The model under review builds one solid part; all positions refer to its coordinate system, in mm. Coordinates: 2 decimals unless noted, no trailing zeros. Loops run counter-clockwise (first coordinate to the right, second up) from the corner with the lowest first, then second, coordinate; pieces in that order, holes last. Notation, with made-up numbers: (57.25, 52.25) - (111.25, 52.25) arc R30 cw to (111.25, 90.25) - close; hole circle Ø3 at (11.25, 49). An arc over 180 degrees is marked (long way). Answer in a Markdown table with one row per item. Add a question column.
(1) For P1, Ø1.5, axis at y = 1, z = -30.5, coming from the +X side; P2, Ø1, axis at x = -1.5, y = 2.5, coming from the -Z side, all flat-tipped, find the tip position at first contact; note any pin that passes through.
(2) We need section D-D on x = 0. Write out the cut boundary in (y, z), plus the area to 3 significant figures.
(3) We need section B-B on y = 1.7. Give the number of separate pieces and of enclosed holes in the cut face, plus the area to 3 significant figures.
(4) We need section C-C on z = 9. Write out the cut boundary in (x, y).
(5) For line 1 along X through (y, z) = (2.1, 0); line 2 along X through (y, z) = (1.9, 30); line 3 along Z through (x, y) = (-32, 1.55), list the stretches that pass through material, from the lowest coordinate up.
(6) Mouldability with a two-part tool opening along X and no side actions: class faces 1 (the cylindrical face through (15.02, 1.48, 47.69)), 2 (the cylindrical face through (-20.196, 1.479, -0.488)), 3 (the flat face through (12, 3, -1)) as +X half, -X half, draft (parallel to the pull), parting line (faces both ways), or undercut.
(7) We need section A-A on x = 30. Write out the cut boundary in (y, z).
from build123d import *

# Parameters (mm, degrees)
SKETCH_1_R          = 50
EXTRUDE_2_DEPTH     = 3
SKETCH_3_R          = 2.25
CUT_EXTRUDE_1_DEPTH = 71.774289117
SKETCH_4_R          = 11
CUT_EXTRUDE_2_DEPTH = 71.774289117


with BuildPart() as part:
    # 草图1 → 凸台-拉伸2 (new body)
    with BuildSketch(Plane(origin=(0, 0, 0), x_dir=(1, 0, 0), z_dir=(0, 1, 0))):
        with Locations(Location((0, 0, 0), (0, 0, 270))):
            Circle(SKETCH_1_R)
    extrude(amount=EXTRUDE_2_DEPTH)

    # 草图3 → 切除-拉伸1 (cut, through all)
    with BuildSketch(Plane(origin=(0, 0, 0), x_dir=(1, 0, 0), z_dir=(0, 1, 0))):
        with Locations(Location((-18, 0, 0), (0, 0, 270))):
            Circle(SKETCH_3_R)
        with Locations(Location((-30, 30, 0), (0, 0, 270))):
            Circle(SKETCH_3_R)
        with Locations(Location((30, 30, 0), (0, 0, 270))):
            Circle(SKETCH_3_R)
        with Locations(Location((30, -30, 0), (0, 0, 270))):
            Circle(SKETCH_3_R)
        with Locations(Location((-30, -30, 0), (0, 0, 270))):
            Circle(SKETCH_3_R)
        with Locations(Location((0, 18, 0), (0, 0, 270))):
            Circle(SKETCH_3_R)
        with Locations(Location((18, 0, 0), (0, 0, 270))):
            Circle(SKETCH_3_R)
        with Locations(Location((0, -18, 0), (0, 0, 270))):
            Circle(SKETCH_3_R)
    extrude(amount=CUT_EXTRUDE_1_DEPTH, mode=Mode.SUBTRACT)

    # 草图4 → 切除-拉伸2 (cut, through all)
    with BuildSketch(Plane(origin=(0, 0, 0), x_dir=(1, 0, 0), z_dir=(0, 1, 0))):
        with Locations(Location((0, 0, 0), (0, 0, 270))):
            Circle(SKETCH_4_R)
    extrude(amount=CUT_EXTRUDE_2_DEPTH, mode=Mode.SUBTRACT)


solid = part.part
Outcome:
| question | item | result |
|---|---|---|
| 1 | P1 | x = 40.19 |
| 1 | P2 | z = -49.99 |
| 2 | outline | (0, -50) - (3, -50) - (3, -20.25) - (0, -20.25) - close; (0, -15.75) - (3, -15.75) - (3, -11) - (0, -11) - close; (0, 11) - (3, 11) - (3, 15.75) - (0, 15.75) - close; (0, 20.25) - (3, 20.25) - (3, 50) - (0, 50) - close |
| 2 | area | 207 mm² |
| 3 | separate pieces | 1 |
| 3 | enclosed holes | 9 |
| 3 | area | 7,350 mm² |
| 4 | outline | (-49.18, 0) - (-6.32, 0) - (-6.32, 3) - (-49.18, 3) - close; (6.32, 0) - (49.18, 0) - (49.18, 3) - (6.32, 3) - close |
| 5 | line 1 | -50 to -20.25, -15.75 to -11, 11 to 15.75, 20.25 to 50 |
| 5 | line 2 | -40 to -32.25, -27.75 to 27.75, 32.25 to 40 |
| 5 | line 3 | -38.42 to -31.03, -28.97 to 28.97, 31.03 to 38.42 |
| 6 | face 1 | parting line |
| 6 | face 2 | undercut |
| 6 | face 3 | draft |
| 7 | outline | (0, -40) - (3, -40) - (3, -32.25) - (0, -32.25) - close; (0, -27.75) - (3, -27.75) - (3, 27.75) - (0, 27.75) - close; (0, 32.25) - (3, 32.25) - (3, 40) - (0, 40) - close |
